The drawing under review shows one solid part. Ordinate dimensions are in mm from its lowest x, y, z. A direction names the side the tool comes from. Give positions to 0.01 mm unless a question says otherwise; leave off trailing zeros. Order: outer loops, then holes, each group sorted by start corner. A loop starts at its lowest first (then second) coordinate and runs counter-clockwise, first axis right, second up. Notation, with made-up numbers: (-40, 14) - (10, 14) arc R16 ccw to (10, 25) - close; hole circle Ø8 at (-33, -32). An arc over 180 degrees is marked (long way). Answer as a JSON object with one key per item and string values. Group by question number.
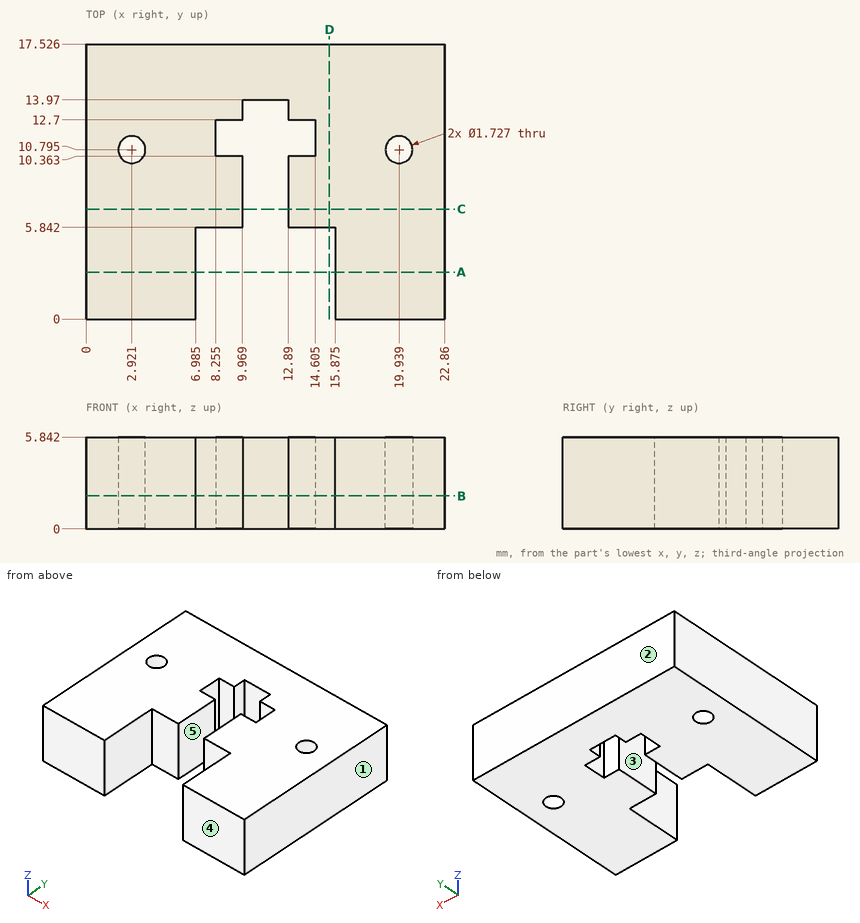
1) For the marked faces 4 and 5, list the 3-axis set-ups (+Z, -Z, +X, -X, +Y, -Y) from which the entire face can be reached by the end or side of a thin tool; tool diameter is ignored.
2) Consider section B-B (z = 2.1). Give the boundary of the cut face in (x, y) (1 decimal), plus the area to 3 significant figures.
3) For pin 1 (1.4 mm diameter, centred on x = 13.5, z = 2.5, fed in from -Y); pin 2 (1.4 mm diameter, centred on x = 2.921, y = 10.795, fed in from -Z), all flat-tipped, find the tip position at first contact; note any pin that passes through.
4) Mouldability with a two-part tool opening along X and no side actions: class the marked faces 1, 2 and 3 as released by +X, released by -X, zero draft, split by the parting line, or undercut.
5) Consider section A-A (y = 3). Give the boundary of the cut face in (x, z) (1 decimal).
6) For line 1 (X direction, y = 4.75, z = 5.2) (1 decimal); line 2 (X direction, y = 7.75, z = 0.4); line 3 (X direction, y = 10.75, z = 2.1) (1 decimal), list the stretches that pass through material, from the lowest coordinate up.
7) Consider section C-C (y = 7). Give the boundary of the cut face in (x, z).
8) Consider section D-D (x = 15.5). Give the boundary of the cut face in (y, z) (1 decimal).
Result set:
{
 "1": {"face 4": "+Z, -Z, +X, -X, -Y", "face 5": "+Z, -Z, -Y"},
 "2": {"outline": "(0, 0) - (7, 0) - (7, 5.8) - (10, 5.8) - (10, 10.4) - (8.3, 10.4) - (8.3, 12.7) - (10, 12.7) - (10, 14) - (12.9, 14) - (12.9, 12.7) - (14.6, 12.7) - (14.6, 10.4) - (12.9, 10.4) - (12.9, 5.8) - (15.9, 5.8) - (15.9, 0) - (22.9, 0) - (22.9, 17.5) - (0, 17.5) - close; hole circle Ø1.7 at (2.9, 10.8); hole circle Ø1.7 at (19.9, 10.8)", "area": "312 mm2"},
 "3": {"pin 1": "stops at y = 5.84", "pin 2": "passes through"},
 "4": {"face 1": "released by +X", "face 2": "zero draft", "face 3": "undercut"},
 "5": {"outline": "(0, 0) - (7, 0) - (7, 5.8) - (0, 5.8) - close; (15.9, 0) - (22.9, 0) - (22.9, 5.8) - (15.9, 5.8) - close"},
 "6": {"line 1": "x = 0 to 7, 15.9 to 22.9", "line 2": "x = 0 to 9.97, 12.89 to 22.86", "line 3": "x = 0 to 2.1, 3.8 to 8.3, 14.6 to 19.1, 20.8 to 22.9"},
 "7": {"outline": "(0, 0) - (9.97, 0) - (9.97, 5.84) - (0, 5.84) - close; (12.89, 0) - (22.86, 0) - (22.86, 5.84) - (12.89, 5.84) - close"},
 "8": {"outline": "(5.8, 0) - (17.5, 0) - (17.5, 5.8) - (5.8, 5.8) - close"}
}
